Autodesk Inventor part; units mm, degrees
ref_plane "YZ Plane" through (0, 0, 0) normal (1, 0, 0) x (0, 1, 0)
ref_plane "XZ Plane" through (0, 0, 0) normal (0, 1, 0) x (-1, 0, 0)
ref_plane "XY Plane" through (0, 0, 0) normal (0, 0, 1) x (1, 0, 0)
sketch "Sketch1" plane through (0, 0, 0) normal (0, 1, 0) x (-1, 0, 0)
  line L0 (0, 0) -> (0, -4.826)
  line L1 (0, -4.826) -> (9.652, -4.826)
  line L2 (9.652, -4.826) -> (9.652, 0)
  line L3 (9.652, 0) -> (0, 0)
  dimension "d0" = 4.826
  dimension "d1" = 9.652
extrude "Extrusion1" add sketch "Sketch1" along normal blind 76.2
fillet "Fillet1" radius 2 2 edges at (0, 38.1, 0) (0, 38.1, -4.826)
sketch "Sketch2" plane through (-9.652, 0, -4.826) normal (-1, 0, 0) x (0, 0, 1)
  line L0 (4.826, 0) -> (4.826, 76.2)
  line L1 (0, 0) -> (0, 76.2)
  line L2 (0, 0) -> (4.826, 0)
  line L3 (0, 76.2) -> (4.826, 76.2)
extrude "Extrusion2" add sketch "Sketch2" along normal blind 1
fillet "Fillet2" radius 1 2 edges at (-10.652, 38.1, -4.826) (-10.652, 38.1, 0)
properties part number "GuideArm"
Source: CAD feature listing. Evaluate the final solid. Frame: model axes, mm. Round coordinates to 2 decimals unless told otherwise and drop trailing zeros. Loops run counter-clockwise (first coordinate to the right, second up) from the corner with the lowest first, then second, coordinate; pieces in that order, holes last.
(1) Material intervals for probe 1 along Z at (x, y) = (-9.75, 8.5); probe 2 along X at (y, z) = (61.5, -1.9); probe 3 along X at (y, z) = (23, -3.6), sorted ascending.
From the geometry:
probe 1: z = -4.82 to 0
probe 2: x = -10.65 to 0
probe 3: x = -10.65 to -0.16
(2) Contact query for a flat-ended pin moving along its axis: pin 1 Ø2 at (x, y) = (-3.5, 65) entering from +Z. Output: stop coordinate, or through.
From the geometry:
pin 1: stops at z = 0
(3) Section query A-A (y = 51.5). Output: boundary loops of the cut face in (x, z).
From the geometry:
outline: (-10.65, -3.83) arc R1 ccw to (-9.65, -4.83) - (-2, -4.83) arc R2 ccw to (0, -2.83) - (0, -2) arc R2 ccw to (-2, 0) - (-9.65, 0) arc R1 ccw to (-10.65, -1) - close
